Input: part model. Units: mm. Frame: model coordinates. Face numbers are marked on the shaded views. A direction names the side the tool comes from. Coordinates: 2 decimals unless noted, no trailing zeros. Order: outer loops, then holes, each group sorted by start corner. A loop starts at its lowest first (then second) coordinate and runs counter-clockwise, first axis right, second up. Notation, with made-up numbers: M 23,51.25 L 41,51.25 A14 ccw 41,56.25 Z; hole C 69,1.25 d2. An arc over 180 degrees is marked long. Answer in a Markdown table with one row per item.
from build123d import *

# Parameters (mm, degrees)
F_12_24_TAPPED_HOLE1_D           = 4.4958
F_12_24_TAPPED_HOLE1_DEPTH       = 19.05
F_12_24_TAPPED_HOLE1_CSINK_D     = 6.7564
F_12_24_TAPPED_HOLE1_CSINK_ANGLE = 82
F_12_24_TAPPED_HOLE1_TIP         = 1.350674586


with BuildPart() as part:
    # Sketch3 → Revolve1 (revolve)
    with BuildSketch(Plane(origin=(0, 0, 0), x_dir=(1, 0, 0), z_dir=(0, 1, 0)), mode=Mode.PRIVATE) as revolve1_sk:
        Polygon((-22.600524836, 0), (25.151475164, 0), (25.151475164, 6.35), (6.101475164, 6.35), (6.101475164, 9.652), (-8.122524836, 9.652), (-8.122524836, 12.7), (-22.600524836, 12.7), align=None)
    revolve(revolve1_sk.sketch.rotate(Axis((-22.600524836, 0, 0), (1, 0, 0)), 180), axis=Axis((-22.600524836, 0, 0), (1, 0, 0)))

    # #12-24 Tapped Hole1
    with Locations(Plane(origin=(25.151475164, 0, 0), x_dir=(0, 0, -1), z_dir=(1, 0, 0))):
        with Locations((0, 0)):
            CounterSinkHole(F_12_24_TAPPED_HOLE1_D / 2, F_12_24_TAPPED_HOLE1_CSINK_D / 2, depth=F_12_24_TAPPED_HOLE1_DEPTH, counter_sink_angle=F_12_24_TAPPED_HOLE1_CSINK_ANGLE)
            with Locations((0, 0, -(F_12_24_TAPPED_HOLE1_DEPTH + F_12_24_TAPPED_HOLE1_TIP / 2))):  # 118° drill point
                Cone(0, F_12_24_TAPPED_HOLE1_D / 2, F_12_24_TAPPED_HOLE1_TIP, mode=Mode.SUBTRACT)


solid = part.part
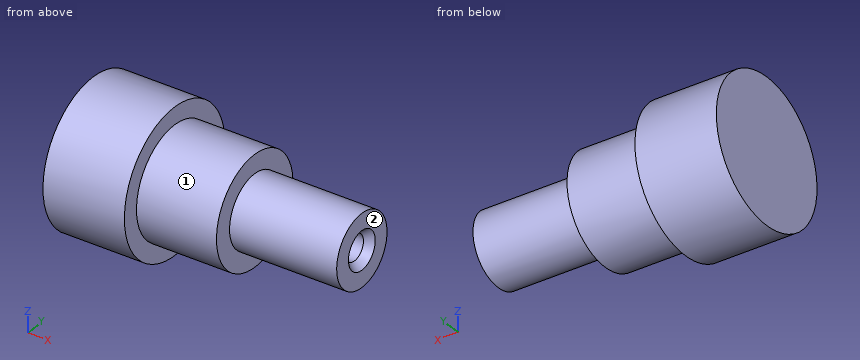
1) Cut plane B-B, the plane z = -4.5. Output: boundary loops of the cut face in (x, y), and give its area (3 significant figures).
Resolved:
| item | result |
|---|---|
| outline | M -22.6,-11.88 L -8.12,-11.88 L -8.12,-8.54 L 6.1,-8.54 L 6.1,-4.48 L 25.15,-4.48 L 25.15,4.48 L 6.1,4.48 L 6.1,8.54 L -8.12,8.54 L -8.12,11.88 L -22.6,11.88 Z |
| area | 757 mm2 |
2) Contact query for flat-ended pins moving along their axis: pin 1 (3 mm diameter, centred on x = -17, y = -8.5, fed in from +Z); pin 2 (5 mm diameter, centred on x = -12, z = 8.5, fed in from -Y); pin 3 (1 mm diameter, centred on x = 18, y = -4.5, fed in from +Z); pin 4 (12.5 mm diameter, centred on y = 2, z = 0, fed in from +X). Output: stop coordinate, or through.
Resolved:
| item | result |
|---|---|
| pin 1 | stops at z = 10.6 |
| pin 2 | stops at y = -11.19 |
| pin 3 | stops at z = 4.93 |
| pin 4 | stops at x = 25.15 |
3) Reachability of the marked faces 1 and 2 from +Z, -Z, +X, -X, +Y, -Y: full face, straight path, thin tool, end or side. Return the list, or none.
Resolved:
| item | result |
|---|---|
| face 1 | +X |
| face 2 | +Z, -Z, +X, +Y, -Y |
4) Cut plane A-A, the plane x = 9. Output: boundary loops of the cut face in (y, z).
Resolved:
| item | result |
|---|---|
| outline | C 0,0 d12.7; hole C 0,0 d4.5 |
5) Cut plane D-D, the plane x = 2. Output: boundary loops of the cut face in (y, z).
Resolved:
| item | result |
|---|---|
| outline | C 0,0 d19.3 |
6) Material intervals for probe 1 along Y at (x, z) = (15.25, 0); probe 2 along X at (y, z) = (-8.5, -3); probe 3 along Y at (x, z) = (-12, 11), sorted ascending.
Resolved:
| item | result |
|---|---|
| probe 1 | y = -6.35 to -2.25, 2.25 to 6.35 |
| probe 2 | x = -22.6 to 6.1 |
| probe 3 | y = -6.35 to 6.35 |
7) Cut plane C-C, the plane x = -13.5. Output: boundary loops of the cut face in (y, z), and give its area (3 significant figures).
Resolved:
| item | result |
|---|---|
| outline | C 0,0 d25.4 |
| area | 507 mm2 |
